Verification items for this drawing (mm, ordinates from the low corner). Coordinates: 2 decimals unless noted, no trailing zeros. Order: outer loops, then holes, each group sorted by start corner. A loop starts at its lowest first (then second) coordinate and runs counter-clockwise, first axis right, second up.
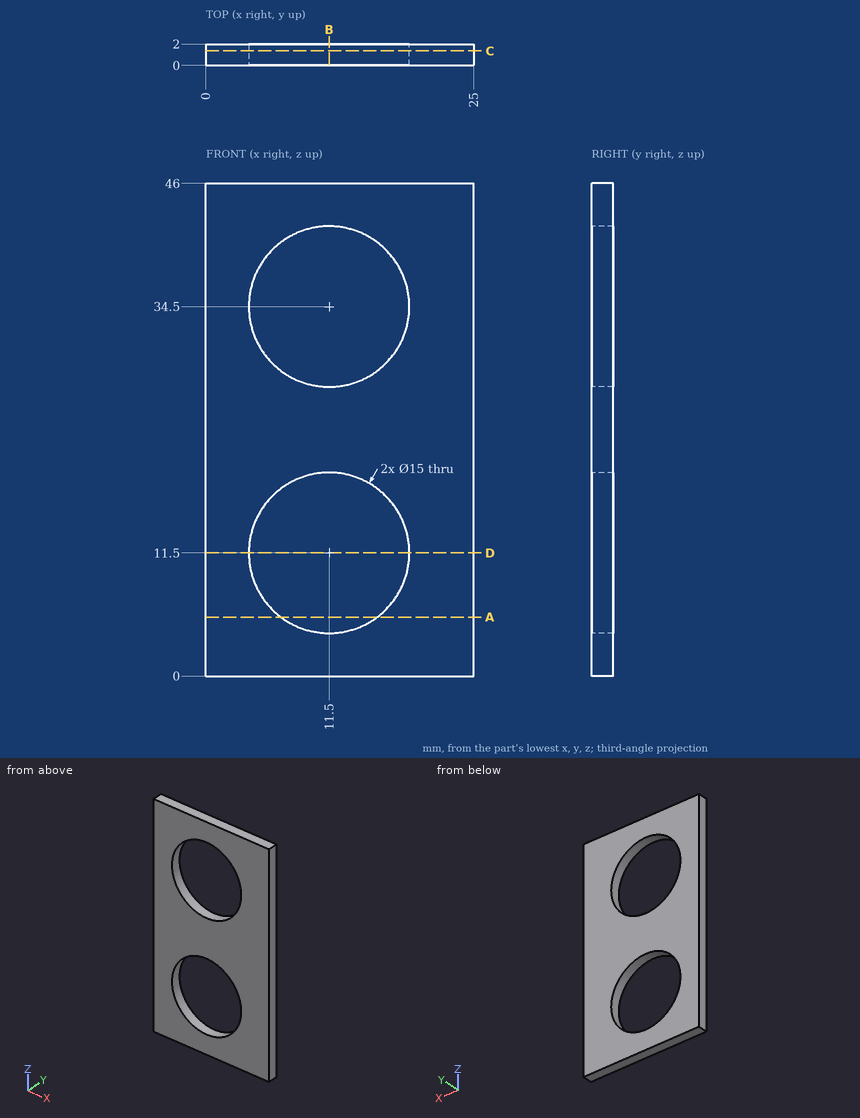
(1) Cross-section at A-A (z = 5.5). Enter the section's corners in (x, y).
Filled in:
outline: (0, 0) - (7, 0) - (7, 2) - (0, 2) - close; (16, 0) - (25, 0) - (25, 2) - (16, 2) - close
(2) Thickness scan on probe 1 along Z at (x, y) = (11.5, 1.65); probe 2 along Z at (x, y) = (8, 1.55); probe 3 along X at (y, z) = (0.5, 12.5). Record the ranges inside material, lowest first.
Filled in:
probe 1: z = 0 to 4, 19 to 27, 42 to 46
probe 2: z = 0 to 4.87, 18.13 to 27.87, 41.13 to 46
probe 3: x = 0 to 4.07, 18.93 to 25
(3) Cross-section at B-B (x = 11.5). Enter the section's corners in (y, z).
Filled in:
outline: (0, 0) - (2, 0) - (2, 4) - (0, 4) - close; (0, 19) - (2, 19) - (2, 27) - (0, 27) - close; (0, 42) - (2, 42) - (2, 46) - (0, 46) - close
(4) Cross-section at D-D (z = 11.5). Enter the section's corners in (x, y).
Filled in:
outline: (0, 0) - (4, 0) - (4, 2) - (0, 2) - close; (19, 0) - (25, 0) - (25, 2) - (19, 2) - close
(5) Cross-section at C-C (y = 1.35). Enter the section's corners in (x, z), and give its area (3 significant figures).
Filled in:
outline: (0, 0) - (25, 0) - (25, 46) - (0, 46) - close; hole circle Ø15 at (11.5, 11.5); hole circle Ø15 at (11.5, 34.5)
area: 797 mm2
(6) Go/stop test with a flat-tipped pin: P1, Ø9, axis at x = 11.5, z = 11.5, coming from the -Y side (1 decimal). Record where the tip stops, or that it passes through.
Filled in:
P1: passes through
